Geometry check sheet. Reference: the model listing, model coordinates, mm. Round coordinates to 2 decimals unless told otherwise and drop trailing zeros. Write each loop counter-clockwise with the first axis right and the second up, starting at its lowest first coordinate (ties: lowest second). Pieces come first, ordered by that corner, then holes. Notation, with made-up numbers: (25.5, -19) - (39.5, -19) arc R22 ccw to (39.5, 18) - close; hole circle Ø11 at (2, -5). An arc over 180 degrees is marked (long way). One line per question, with ' | ' between items. Start each with the question number.
from build123d import *

# Parameters (mm, degrees)
BOSS_EXTRU_1_DEPTH       = 2.5
ESQUISSE22_R             = 12.6
ENL_V_MAT_EXTRU_1_DEPTH  = 2.5
ESQUISSE23_R             = 3
ENL_V_MAT_EXTRU_2_DEPTH  = 2.5
ENL_V_MAT_EXTRU_3_DEPTH  = 2.5
ESQUISSE25_W             = 13
ESQUISSE25_H             = 3.371774097
ENL_V_MAT_EXTRU_4_DEPTH  = 2.5
CONG_1_R                 = 2
ESQUISSE26_R             = 6.5
ENL_V_MAT_EXTRU_5_DEPTH  = 2.5
ESQUISSE27_R             = 6.5
ENL_V_MAT_EXTRU_6_DEPTH  = 2.5
ESQUISSE30_W             = 13
ESQUISSE30_H             = 3.36
ENL_V_MAT_EXTRU_7_DEPTH  = 2.5
CONG_2_R                 = 2
ESQUISSE31_R             = 3
ENL_V_MAT_EXTRU_8_DEPTH  = 2.5
ENL_V_MAT_EXTRU_9_DEPTH  = 2.5
ESQUISSE33_R             = 3
ENL_V_MAT_EXTRU_10_DEPTH = 10
ESQUISSE34_R             = 3
ENL_V_MAT_EXTRU_11_DEPTH = 10


with BuildPart() as part:
    # Esquisse20 → Boss.-Extru.1 (new body)
    with BuildSketch(Plane.XY):
        with BuildLine():
            Line((14.8, -2), (164.37, -2))
            ThreePointArc((164.37, -2), (174.835180362, 2.334819638), (179.17, 12.8))
            Line((179.17, 12.8), (179.17, 57.73))
            ThreePointArc((179.17, 57.73), (177.851980515, 60.911980515), (174.67, 62.23))
            Line((174.67, 62.23), (4.5, 62.23))
            ThreePointArc((4.5, 62.23), (1.318019485, 60.911980515), (0, 57.73))
            Line((0, 57.73), (0, 12.8))
            ThreePointArc((0, 12.8), (4.334819638, 2.334819638), (14.8, -2))
        make_face()
    extrude(amount=BOSS_EXTRU_1_DEPTH)

    # Esquisse22 → Enlèv. mat.-Extru.1 (cut)
    with BuildSketch(Plane.XY.offset(2.5)):
        with Locations((26.77, 24.77)):
            Circle(ESQUISSE22_R)
    extrude(amount=-ENL_V_MAT_EXTRU_1_DEPTH, mode=Mode.SUBTRACT)

    # Esquisse23 → Enlèv. mat.-Extru.2 (cut)
    with BuildSketch(Plane.XY.offset(2.5)):
        with Locations((8.99, 13.97)):
            Circle(ESQUISSE23_R)
    extrude(amount=-ENL_V_MAT_EXTRU_2_DEPTH, mode=Mode.SUBTRACT)

    # Esquisse24 → Enlèv. mat.-Extru.3 (cut)
    with BuildSketch(Plane.XY.offset(2.5)):
        Polygon((36.78, 58.87), (36.78, 50.15), (49.78, 50.15), align=None)
        Polygon((49.78, 58.87), (49.78, 50.15), (36.78, 58.87), align=None)
    extrude(amount=-ENL_V_MAT_EXTRU_3_DEPTH, mode=Mode.SUBTRACT)

    # Esquisse25 → Enlèv. mat.-Extru.4 (cut)
    with BuildSketch(Plane.XY.offset(2.5)):
        with Locations((43.28, 60.555887049)):
            Rectangle(ESQUISSE25_W, ESQUISSE25_H)
    extrude(amount=-ENL_V_MAT_EXTRU_4_DEPTH, mode=Mode.SUBTRACT)

    # Congé1
    cong_1_edges = [part.edges().sort_by_distance(p)[0] for p in [
        (49.78, 62.23, 1.25),
        (36.78, 62.23, 1.25),
    ]]
    fillet(cong_1_edges, radius=CONG_1_R)

    # Esquisse26 → Enlèv. mat.-Extru.5 (cut)
    with BuildSketch(Plane.XY.offset(2.5)):
        with Locations((156.21, 22.13)):
            Circle(ESQUISSE26_R)
    extrude(amount=-ENL_V_MAT_EXTRU_5_DEPTH, mode=Mode.SUBTRACT)

    # Esquisse27 → Enlèv. mat.-Extru.6 (cut)
    with BuildSketch(Plane.XY.offset(2.5)):
        with Locations((146.05, 11.97)):
            Circle(ESQUISSE27_R)
        with Locations((135.89, 22.13)):
            Circle(ESQUISSE27_R)
        with Locations((146.05, 31.65)):
            Circle(ESQUISSE27_R)
    extrude(amount=-ENL_V_MAT_EXTRU_6_DEPTH, mode=Mode.SUBTRACT)

    # Esquisse30 → Enlèv. mat.-Extru.7 (cut)
    with BuildSketch(Plane.XY.offset(2.5)):
        with Locations((135.26, 60.55)):
            Rectangle(ESQUISSE30_W, ESQUISSE30_H)
        Polygon((141.76, 58.87), (128.76, 58.87), (135.26, 54.51), align=None)
        Polygon((135.26, 54.51), (128.76, 58.87), (128.76, 50.15), align=None)
        Polygon((141.76, 50.15), (135.26, 54.51), (128.76, 50.15), align=None)
        Polygon((141.76, 58.87), (135.26, 54.51), (141.76, 50.15), align=None)
    extrude(amount=-ENL_V_MAT_EXTRU_7_DEPTH, mode=Mode.SUBTRACT)

    # Congé2
    cong_2_edges = [part.edges().sort_by_distance(p)[0] for p in [
        (128.76, 62.23, 1.25),
        (141.76, 62.23, 1.25),
    ]]
    fillet(cong_2_edges, radius=CONG_2_R)

    # Esquisse31 → Enlèv. mat.-Extru.8 (cut)
    with BuildSketch(Plane.XY.offset(2.5)):
        with Locations((147.96, 54.51)):
            Circle(ESQUISSE31_R)
        with Locations((139.7, 44.99)):
            Circle(ESQUISSE31_R)
    extrude(amount=-ENL_V_MAT_EXTRU_8_DEPTH, mode=Mode.SUBTRACT)

    # Esquisse32 → Enlèv. mat.-Extru.9 (cut)
    with BuildSketch(Plane.XY.offset(2.5)):
        with BuildLine():
            Line((172.018614708, 50.217190958), (155.048051959, 44.217190958))
            ThreePointArc((155.048051959, 44.217190958), (153.771909584, 44.826666667), (154.381385292, 46.102809042))
            Line((154.381385292, 46.102809042), (171.351948041, 52.102809042))
            ThreePointArc((171.351948041, 52.102809042), (172.628090416, 51.493333333), (172.018614708, 50.217190958))
        make_face()
        with BuildLine():
            Line((153.866666667, 49.102809042), (169.866666667, 54.759663291))
            ThreePointArc((169.866666667, 54.759663291), (171.142809042, 54.150187583), (170.533333333, 52.874045208))
            Line((170.533333333, 52.874045208), (154.533333333, 47.217190958))
            ThreePointArc((154.533333333, 47.217190958), (153.257190958, 47.826666667), (153.866666667, 49.102809042))
        make_face()
        with BuildLine():
            Line((154.542111346, 52.523595314), (167.191221987, 56.995731269))
            ThreePointArc((167.191221987, 56.995731269), (168.467364362, 56.38625556), (167.857888654, 55.110113185))
            Line((167.857888654, 55.110113185), (155.208778013, 50.63797723))
            ThreePointArc((155.208778013, 50.63797723), (153.932635638, 51.247452939), (154.542111346, 52.523595314))
        make_face()
        with BuildLine():
            Line((155.866666667, 43.445954792), (171.866666667, 49.102809042))
            ThreePointArc((171.866666667, 49.102809042), (173.142809042, 48.493333333), (172.533333333, 47.217190958))
            Line((172.533333333, 47.217190958), (156.533333333, 41.560336709))
            ThreePointArc((156.533333333, 41.560336709), (155.257190958, 42.169812417), (155.866666667, 43.445954792))
        make_face()
        with BuildLine():
            Line((158.617948097, 41.177385778), (171.09857492, 45.446217537))
            ThreePointArc((171.09857492, 45.446217537), (172.368388344, 44.823663229), (171.745834035, 43.553849804))
            Line((171.745834035, 43.553849804), (159.265207213, 39.285018045))
            ThreePointArc((159.265207213, 39.285018045), (157.995393788, 39.907572354), (158.617948097, 41.177385778))
        make_face()
    extrude(amount=-ENL_V_MAT_EXTRU_9_DEPTH, mode=Mode.SUBTRACT)

    # Esquisse33 → Enlèv. mat.-Extru.10 (cut)
    with BuildSketch(Plane.XY.offset(2.5)):
        with Locations((38.83, 44.99)):
            Circle(ESQUISSE33_R)
    extrude(amount=-ENL_V_MAT_EXTRU_10_DEPTH, mode=Mode.SUBTRACT)

    # Esquisse34 → Enlèv. mat.-Extru.11 (cut)
    with BuildSketch(Plane.XY.offset(2.5)):
        with Locations((10.26, 4.99)):
            Circle(ESQUISSE34_R)
    extrude(amount=-ENL_V_MAT_EXTRU_11_DEPTH, mode=Mode.SUBTRACT)


solid = part.part
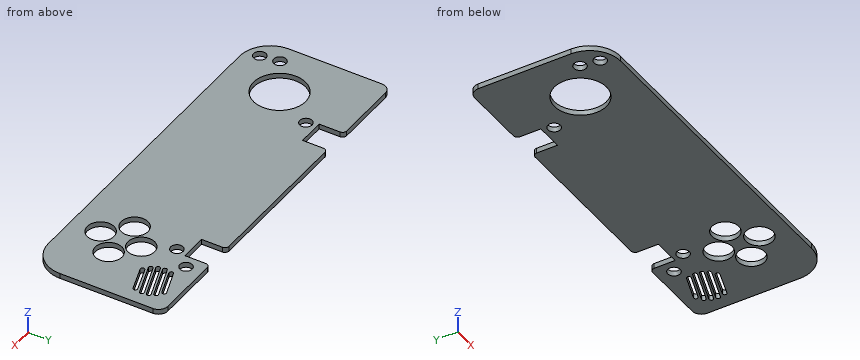
Q1. Thickness scan on line 1 (Y direction, x = 140.5, z = 0.95); line 2 (Y direction, x = 147.96, z = 1.2); line 3 (X direction, y = 6.5, z = 0.45). Record the ranges inside material, lowest first.
Q2. Go/stop test with flat-tipped pins: P1, Ø8, axis at x = 135.89, y = 22.13, coming from the -Z side; P2, Ø0.8, axis at x = 45, z = 0.5, coming from the +Y side. Record where each tip stops, or that it passes through.
Q3. Section check A-A, the plane y = 22.13. Record the cut outline in (x, z).
Q4. Section check B-B, the plane z = 1.2. Count the separate pieces of the cut face and the enclosed holes in it, then the cut area to 3 significant figures.
Result sheet:
1) line 1: -2 to 8.59, 15.35 to 17.55, 26.71 to 28.27, 35.03 to 42.1, 47.88 to 50.15 | line 2: -2 to 5.76, 18.18 to 25.44, 37.86 to 51.51, 57.51 to 62.23 | line 3: 1.41 to 7.67, 12.85 to 142.54, 149.56 to 177.76
2) P1: through | P2: y = 50.15
3) outline: (0, 0) - (14.45, 0) - (14.45, 2.5) - (0, 2.5) - close; (39.09, 0) - (129.39, 0) - (129.39, 2.5) - (39.09, 2.5) - close; (142.39, 0) - (149.71, 0) - (149.71, 2.5) - (142.39, 2.5) - close; (162.71, 0) - (179.17, 0) - (179.17, 2.5) - (162.71, 2.5) - close
4) separate pieces: 1 | enclosed holes: 15 | area: 9,740 mm²
